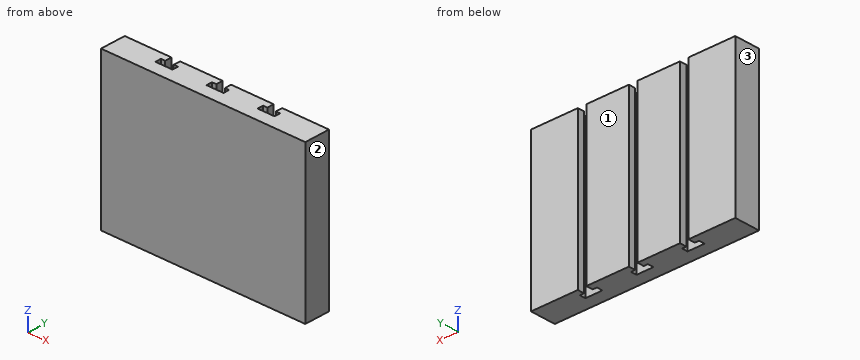
```python
from build123d import *

# Parameters (mm, degrees)
SKETCH3_W           = 120
SKETCH3_H           = 15
BOSS_EXTRUDE2_DEPTH = 90
CUT_EXTRUDE1_DEPTH  = 90


with BuildPart() as part:
    # Sketch3 → Boss-Extrude2 (new body)
    with BuildSketch(Plane.XY):
        Rectangle(SKETCH3_W, SKETCH3_H)
    extrude(amount=BOSS_EXTRUDE2_DEPTH)

    # Sketch6 → Cut-Extrude1 (cut)
    with BuildSketch(Plane.XY.offset(90)):
        Polygon((32.5, 3.5), (35, 3.5), (35, 0), (25, 0), (25, 3.5), (27.5, 3.5), (27.5, 7.5), (32.5, 7.5), align=None)
        Polygon((-27.5, 3.5), (-25, 3.5), (-25, 0), (-35, 0), (-35, 3.5), (-32.5, 3.5), (-32.5, 7.5), (-27.5, 7.5), align=None)
        Polygon((-2.5, 7.5), (2.5, 7.5), (2.5, 3.5), (5, 3.5), (5, 0), (-5, 0), (-5, 3.5), (-2.5, 3.5), align=None)
    extrude(amount=-CUT_EXTRUDE1_DEPTH, mode=Mode.SUBTRACT)


solid = part.part
```
Model file for the job. Use its own axes, mm. Face numbers are marked on the shaded views. Coordinates: 2 decimals unless noted, no trailing zeros. Order: outer loops, then holes, each group sorted by start corner. A loop starts at its lowest first (then second) coordinate and runs counter-clockwise, first axis right, second up. Notation, with made-up numbers: (80.25, 33) -> (85.25, 33) arc R31 cw to (85.25, 65) -> close; hole circle Ø3 at (39, 80.5). An arc over 180 degrees is marked (long way). Answer as a JSON object with one key per item and string values. Group by question number.
1) Pull direction X, two halves, no side cores. Call the marked faces 1, 2 and 3: +X half, -X half, draft (parallel to the pull), parting line (faces both ways), or undercut.
2) Cut at B-B, the plane x = -29.5. Write the cut outline in (y, z), then the cut area to 3 significant figures.
3) Cut at A-A, the plane z = 15.5. Write the cut outline in (x, y), then the cut area to 4 significant figures.
4) Drill centre lines: L1, parallel to X at y = 4.25, z = 77; L2, parallel to X at y = 0.5, z = 82.5; L3, parallel to Y at x = 3, z = 82.5. Where is each one in solid material? Low to high.
Check values:
{
 "1": {"face 1": "draft", "face 2": "+X half", "face 3": "-X half"},
 "2": {"outline": "(-7.5, 0) -> (0, 0) -> (0, 90) -> (-7.5, 90) -> close", "area": "675 mm²"},
 "3": {"outline": "(-60, -7.5) -> (60, -7.5) -> (60, 7.5) -> (32.5, 7.5) -> (32.5, 3.5) -> (35, 3.5) -> (35, 0) -> (25, 0) -> (25, 3.5) -> (27.5, 3.5) -> (27.5, 7.5) -> (2.5, 7.5) -> (2.5, 3.5) -> (5, 3.5) -> (5, 0) -> (-5, 0) -> (-5, 3.5) -> (-2.5, 3.5) -> (-2.5, 7.5) -> (-27.5, 7.5) -> (-27.5, 3.5) -> (-25, 3.5) -> (-25, 0) -> (-35, 0) -> (-35, 3.5) -> (-32.5, 3.5) -> (-32.5, 7.5) -> (-60, 7.5) -> close", "area": "1,635 mm²"},
 "4": {"L1": "x = -60 to -32.5, -27.5 to -2.5, 2.5 to 27.5, 32.5 to 60", "L2": "x = -60 to -35, -25 to -5, 5 to 25, 35 to 60", "L3": "y = -7.5 to 0, 3.5 to 7.5"}
}
